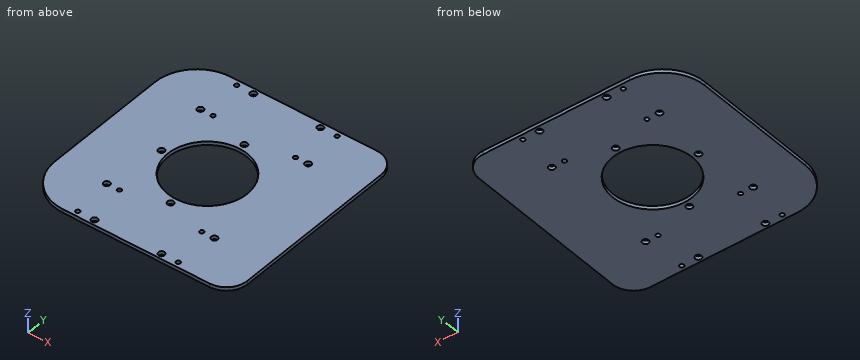
```python
from build123d import *

# Parameters (mm, degrees)
SKETCH_1_W          = 58
SKETCH_1_H          = 100
SKETCH_1_R          = 1
SKETCH_1_R_2        = 1.5
EXTRUDE_1_DEPTH     = 3
SKETCH_2_R          = 1.5
SKETCH_2_R_2        = 19
CUT_EXTRUDE_1_DEPTH = 10
SKETCH_2_3_W        = 20
SKETCH_2_3_H        = 100
SKETCH_2_3_W_2      = 22
EXTRUDE_2_DEPTH     = 3
FILLET_1_R          = 20
FILLET_2_R          = 10
CUT_EXTRUDE_2_DEPTH = 1.3


with BuildPart() as part:
    # Sketch 1 → Extrude 1 (new body)
    with BuildSketch(Plane.XY):
        Rectangle(SKETCH_1_W, SKETCH_1_H)
        with Locations((-24, 47.5)):
            Circle(SKETCH_1_R, mode=Mode.SUBTRACT)
        with Locations((-16, 47.5)):
            Circle(SKETCH_1_R_2, mode=Mode.SUBTRACT)
        with Locations(Location((16, 47.5, 0), (0, 0, 180))):
            Circle(SKETCH_1_R_2, mode=Mode.SUBTRACT)
        with Locations(Location((24, 47.5, 0), (0, 0, 180))):
            Circle(SKETCH_1_R, mode=Mode.SUBTRACT)
        with Locations((-19.7, 28)):
            Circle(SKETCH_1_R, mode=Mode.SUBTRACT)
        with Locations((-25.7, 28)):
            Circle(SKETCH_1_R_2, mode=Mode.SUBTRACT)
        with Locations(Location((19.7, 28, 0), (0, 0, 180))):
            Circle(SKETCH_1_R, mode=Mode.SUBTRACT)
        with Locations(Location((25.7, 28, 0), (0, 0, 180))):
            Circle(SKETCH_1_R_2, mode=Mode.SUBTRACT)
        with Locations((25.7, -28)):
            Circle(SKETCH_1_R_2, mode=Mode.SUBTRACT)
        with Locations((24, -47.5)):
            Circle(SKETCH_1_R, mode=Mode.SUBTRACT)
        with Locations((16, -47.5)):
            Circle(SKETCH_1_R_2, mode=Mode.SUBTRACT)
        with Locations((19.7, -28)):
            Circle(SKETCH_1_R, mode=Mode.SUBTRACT)
        with Locations(Location((-19.7, -28, 0), (0, 0, 180))):
            Circle(SKETCH_1_R, mode=Mode.SUBTRACT)
        with Locations(Location((-25.7, -28, 0), (0, 0, 180))):
            Circle(SKETCH_1_R_2, mode=Mode.SUBTRACT)
        with Locations(Location((-24, -47.5, 0), (0, 0, 180))):
            Circle(SKETCH_1_R, mode=Mode.SUBTRACT)
        with Locations(Location((-16, -47.5, 0), (0, 0, 180))):
            Circle(SKETCH_1_R_2, mode=Mode.SUBTRACT)
    extrude(amount=EXTRUDE_1_DEPTH)

    # Sketch 2 → Cut-Extrude 1 (cut)
    with BuildSketch(Plane.XY.offset(3)):
        with Locations((0, -22)):
            Circle(SKETCH_2_R)
        with Locations((-22, 0)):
            Circle(SKETCH_2_R)
        with Locations((0, 22)):
            Circle(SKETCH_2_R)
        Circle(SKETCH_2_R_2)
    extrude(amount=-CUT_EXTRUDE_1_DEPTH, mode=Mode.SUBTRACT)

    # Sketch 2_3 → Extrude 2 (add)
    with BuildSketch(Plane.XY.offset(3)):
        with Locations((-39, 0)):
            Rectangle(SKETCH_2_3_W, SKETCH_2_3_H)
        with Locations((40, 0)):
            Rectangle(SKETCH_2_3_W_2, SKETCH_2_3_H)
    extrude(amount=-EXTRUDE_2_DEPTH)

    # Fillet 1
    fillet_1_edges = [part.edges().sort_by_distance(p)[0] for p in [
        (-49, -50, 1.5),
        (-49, 50, 1.5),
    ]]
    fillet(fillet_1_edges, radius=FILLET_1_R)

    # Fillet 2
    fillet_2_edges = [part.edges().sort_by_distance(p)[0] for p in [
        (51, 50, 1.5),
        (51, -50, 1.5),
    ]]
    fillet(fillet_2_edges, radius=FILLET_2_R)

    # Sketch 3 → Cut-Extrude 2 (cut)
    with BuildSketch(Plane(origin=(0, 0, 0), x_dir=(-1, 0, 0), z_dir=(0, 0, -1))):
        with BuildLine():
            Line((29, 50), (-41, 50))
            ThreePointArc((-41, 50), (-48.071067812, 47.071067812), (-51, 40))
            Line((-51, 40), (-51, -40))
            ThreePointArc((-51, -40), (-48.071067812, -47.071067812), (-41, -50))
            Line((-41, -50), (29, -50))
            ThreePointArc((29, -50), (43.142135624, -44.142135624), (49, -30))
            Line((49, -30), (49, 30))
            ThreePointArc((49, 30), (43.142135624, 44.142135624), (29, 50))
        make_face()
    extrude(amount=-CUT_EXTRUDE_2_DEPTH, mode=Mode.SUBTRACT)


solid = part.part
```
Check sheet for the modelled part. Datum: model origin and axes. Units: mm. Give positions to 0.01 mm unless a question says otherwise; leave off trailing zeros. Write each loop counter-clockwise with the first axis right and the second up, starting at its lowest first coordinate (ties: lowest second). Pieces come first, ordered by that corner, then holes.
Item 1: Cross-section at B-B (x = 0). Enter the section's corners in (y, z), and give its area (3 significant figures).
Item 2: Cross-section at C-C (z = 2.2). Count the separate pieces of the cut face and the enclosed holes in it, and give its area (3 significant figures).
Item 3: Cross-section at D-D (y = 8.5). Enter the section's corners in (x, z), and give its area (3 significant figures).
Item 4: Scan lines: L1, parallel to Y at x = -25.7, z = 1.7; L2, parallel to X at y = 28, z = 2.45; L3, parallel to Y at x = 16, z = 1.8. Record each from-to range of solid material in increasing order.
Item 5: Cross-section at A-A (y = -22). Enter the section's corners in (x, z), and give its area (3 significant figures).
Item 6: Gauge pin test, flat end, axial feed: pin 1 (1.8 mm diameter, centred on x = 19.7, y = -28, fed in from -Z). Record the tip position at first contact, or that the pin passes through.
Report:
1. outline: (-50, 1.3) - (-23.5, 1.3) - (-23.5, 3) - (-50, 3) - close; (-20.5, 1.3) - (-19, 1.3) - (-19, 3) - (-20.5, 3) - close; (19, 1.3) - (20.5, 1.3) - (20.5, 3) - (19, 3) - close; (23.5, 1.3) - (50, 1.3) - (50, 3) - (23.5, 3) - close
1. area: 95.2 mm2
2. separate pieces: 1
2. enclosed holes: 20
2. area: 8,550 mm2
3. outline: (-49, 1.3) - (-16.99, 1.3) - (-16.99, 3) - (-49, 3) - close; (16.99, 1.3) - (51, 1.3) - (51, 3) - (16.99, 3) - close
3. area: 112 mm2
4. L1: y = -50 to -29.5, -26.5 to 26.5, 29.5 to 50
4. L2: x = -49 to -27.2, -24.2 to -20.7, -18.7 to 18.7, 20.7 to 24.2, 27.2 to 51
4. L3: y = -50 to -49, -46 to -10.25, 10.25 to 46, 49 to 50
5. outline: (-49, 1.3) - (-1.5, 1.3) - (-1.5, 3) - (-49, 3) - close; (1.5, 1.3) - (51, 1.3) - (51, 3) - (1.5, 3) - close
5. area: 165 mm2
6. pin 1: passes through
